Part model, mm, in its own coordinate system. A direction names the side the tool comes from. Round coordinates to 2 decimals unless told otherwise and drop trailing zeros. Write each loop counter-clockwise with the first axis right and the second up, starting at its lowest first coordinate (ties: lowest second). Pieces come first, ordered by that corner, then holes. Notation, with made-up numbers: (55, 28.25) -> (106, 28.25) arc R23 ccw to (106, 57.25) -> close; hole circle Ø4 at (62, 56). An arc over 180 degrees is marked (long way). Return JSON: item names as keys, results as strings. Group by question number.
(1) Saw through at D-D (x = -3). List the corners of the cut face in (y, z).
(2) Tool access for faces 1 (the flat face through (-10, -41, 15)), 2 (the cylindrical face through (-19.86, -3.01, 27.15)), 3 (the flat face through (-15, -40, -10)): list every direction of +Z, -Z, +X, -X, +Y, -Y with a clear straight run to the whole face (end or side of a thin tool).
(3) Saw through at C-C (y = -67). List the corners of the cut face in (x, z), plus the area to 3 significant figures.
(4) Saw through at A-A (z = -10.5). List the corners of the cut face in (x, y).
(5) Drop flat-ended pins along their axis: pin 1 Ø22 at (x, y) = (3.5, -52.5) entering from +Z; pin 2 Ø22 at (x, y) = (-16, -24.5) entering from -Z; pin 3 Ø3 at (y, z) = (-19, 14) entering from +X. Give the stop position or say it passes through.
(6) Saw through at B-B (x = -22). List the corners of the cut face in (y, z).
(7) Drill centre lines: L1, parallel to Z at x = 2, y = -68; L2, parallel to X at y = -65.5, z = 21; L3, parallel to Y at x = -5.5, z = -7. Where is each one in solid material? Low to high. Write a range as from..to.
from build123d import *

# Parameters (mm, degrees)
SKETCH1_W           = 20
SKETCH1_H           = 80
BOSS_EXTRUDE1_DEPTH = 30
SKETCH2_W           = 40
SKETCH2_H           = 40
BOSS_EXTRUDE2_DEPTH = 20
FILLET1_R           = 10


with BuildPart() as part:
    # Sketch1 → Boss-Extrude1 (new body)
    with BuildSketch(Plane.XY):
        with Locations((-20, -40)):
            Rectangle(SKETCH1_W, SKETCH1_H)
    extrude(amount=BOSS_EXTRUDE1_DEPTH)

    # Sketch2 → Boss-Extrude2 (add)
    with BuildSketch(Plane.XY):
        with Locations((-10, -60)):
            Rectangle(SKETCH2_W, SKETCH2_H)
    extrude(amount=-BOSS_EXTRUDE2_DEPTH)

    # Fillet1
    fillet1_edges = [part.edges().sort_by_distance(p)[0] for p in [
        (10, -40, -10),
        (-20, 0, 30),
    ]]
    fillet(fillet1_edges, radius=FILLET1_R)


solid = part.part
Computed values:
{
 "1": {"outline": "(-80, -20) -> (-40, -20) -> (-40, 0) -> (-80, 0) -> close"},
 "2": {"face 1": "+Z, +X, +Y, -Y", "face 2": "+Z, +X, -X, +Y", "face 3": "-Z, +X, -X, +Y"},
 "3": {"outline": "(-30, -20) -> (10, -20) -> (10, 0) -> (-10, 0) -> (-10, 30) -> (-30, 30) -> close", "area": "1,400 mm2"},
 "4": {"outline": "(-30, -80) -> (10, -80) -> (10, -50) arc R10 ccw to (0, -40) -> (-30, -40) -> close"},
 "5": {"pin 1": "z = 0", "pin 2": "z = 0", "pin 3": "x = -10"},
 "6": {"outline": "(-80, -20) -> (-40, -20) -> (-40, 0) -> (0, 0) -> (0, 20) arc R10 ccw to (-10, 30) -> (-80, 30) -> close"},
 "7": {"L1": "-20..0", "L2": "-30..-10", "L3": "-80..-40"}
}
